from build123d import *

# Parameters (mm, degrees)
F0_W     = 11.7
F0_H     = 4
F1_DEPTH = 88.9
F3_DEPTH = 25
F4_R     = 0.5
F5_DEPTH = 25
F6_R     = 1
F7_DEPTH = 12.701
F13_R    = 0.5


with BuildPart() as f1:
    # F0 (on Top) → F1 (new body)
    with BuildSketch(Plane.XY):
        with BuildLine():
            Line((12.2, 0), (0.5, 0))
            ThreePointArc((0.5, 0), (0.1464466094, -0.1464466094), (0, -0.5))
            Line((0, -0.5), (0, -4.5))
            ThreePointArc((0, -4.5), (0.1464466094, -4.8535533906), (0.5, -5))
            Line((0.5, -5), (12.2, -5))
            ThreePointArc((12.2, -5), (12.5535533906, -4.8535533906), (12.7, -4.5))
            Line((12.7, -4.5), (12.7, -0.5))
            ThreePointArc((12.7, -0.5), (12.5535533906, -0.1464466094), (12.2, 0))
        make_face()
        with Locations((6.35, -2.5)):
            Rectangle(F0_W, F0_H, mode=Mode.SUBTRACT)
    extrude(amount=F1_DEPTH)

    # F2 (on face) → F3 (cut)
    with BuildSketch(Plane.XZ.offset(5)):
        Polygon((3.7468838188, 3.0342543032), (1.7641486272, 0), (10.9358513728, 0), (8.9531161812, 3.0342543032), (6.35, 3.0342543032), align=None)
    extrude(amount=-F3_DEPTH, mode=Mode.SUBTRACT)

    # F4 (on face) → F5 (cut)
    with BuildSketch(Plane(origin=(0, 0, 0), x_dir=(-1, 0, 0), z_dir=(0, 1, 0))):
        with Locations((-6.35, 17.8078599274)):
            Circle(F4_R)
    extrude(amount=-F5_DEPTH, mode=Mode.SUBTRACT)

    # F6 (on face) → F7 (cut, through all)
    with BuildSketch(Plane.YZ.offset(12.7)):
        with Locations((-2.5, 17.5)):
            Circle(F6_R)
    extrude(amount=-F7_DEPTH, mode=Mode.SUBTRACT)

    # F9 (on offset) → F10 (revolve)
    with BuildSketch(Plane.XY.offset(17.5)):
        Polygon((0.5120678688, -1.5), (0, -1.5), (0.1683332375, -2.5), (0.6804011064, -2.5), align=None)
    revolve(axis=Axis((0.6804011064, -2.5, 17.5), (1, 0, 0)))

    # F12: F1 across plane


with BuildPart() as f1_1:
    add(f1.part)
    add(f1.part.mirror(Plane(origin=(6.35, -2.5, 44.6902153566), x_dir=(0, 1, 0), z_dir=(1, 0, 0))))

    # F13
    f13_edges = [f1_1.edges().sort_by_distance(p)[0] for p in [
        (12.2, -4.5, 44.45),
        (0.5, -4.5, 44.45),
        (0.5, -0.5, 44.45),
        (12.2, -0.5, 44.45),
    ]]
    fillet(f13_edges, radius=F13_R)


solid = f1_1.part
Check sheet for the modelled part. Datum: model origin and axes. Units: mm. A direction names the side the tool comes from. Give positions to 0.01 mm unless a question says otherwise; leave off trailing zeros. Write each loop counter-clockwise with the first axis right and the second up, starting at its lowest first coordinate (ties: lowest second). Pieces come first, ordered by that corner, then holes. Notation, with made-up numbers: M -39.75,24.25 L -2.75,24.25 A27 ccw -2.75,40.25 Z; hole C 71,-8.75 d11. An arc over 180 degrees is marked long. Use one line per item in the form item = value.
(1) Draft check along Y on faces 1 (the flat face through (9.958, -0.253, 1.496)), 2 (the conical face through (12.03, -2.47, 17.44)), 3 (the flat face through (0.5, -3, 44)), 4 (the flat face through (6, 0, 44)). Enter one of: pulls with the +Y half, pulls with the -Y half, needs draft (parallel to the pull), parting line crosses it, or undercut.
Answer block:
face_1 = needs draft
face_2 = undercut
face_3 = undercut
face_4 = pulls with the +Y half
(2) Section check B-B on x = 10. Record the boundary of the cut face in (y, z).
Answer block:
outline = M -5,1.43 L -4.5,1.43 L -4.5,88.9 L -5,88.9 Z; M -0.5,1.43 L 0,1.43 L 0,88.9 L -0.5,88.9 Z
(3) Section check A-A on z = 15. Record the boundary of the cut face in (x, y).
Answer block:
outline = M 0,-4.5 A0.5 ccw 0.5,-5 L 12.2,-5 A0.5 ccw 12.7,-4.5 L 12.7,-0.5 A0.5 ccw 12.2,0 L 0.5,0 A0.5 ccw 0,-0.5 Z; hole M 0.5,-4 A0.5 ccw 1,-4.5 L 11.7,-4.5 A0.5 ccw 12.2,-4 L 12.2,-1 A0.5 ccw 11.7,-0.5 L 1,-0.5 A0.5 ccw 0.5,-1 Z
(4) Material ranges on line 1 along Z through (x, y) = (6.35, -0.15); line 2 along Y through (x, z) = (9.75, 55.5); line 3 along X through (y, z) = (-3.55, 17), recorded low to high.
Answer block:
line_1 = 3.03 to 17.31, 18.31 to 88.9
line_2 = -5 to -4.5, -0.5 to 0
line_3 = 0 to 0.5, 12.2 to 12.7
(5) Tool access check on faces 5 (the conical face through (0.67, -2.47, 17.44)), 6 (the flat face through (6.3, -4.7, 88.9)), 7 (the flat face through (6, -5, 44)), 8 (the flat face through (6, -4.5, 44)), 9 (the flat face through (9.958, -4.754, 1.496)). Record the directions out of +Z, -Z, +X, -X, +Y, -Y that give a thin tool (end or side, any length) a straight path to the whole face; none if there is none.
Answer block:
face_5 = none
face_6 = +Z, +X, -X, +Y, -Y
face_7 = +Z, -Z, +X, -X, -Y
face_8 = +Z, -Z
face_9 = -Z, +Y, -Y
(6) Depth check by flat-ended pin: P1, Ø3, axis at x = 7.5, y = -4, coming from the -Z side. Enter the tip coordinate at first touch or a pass-through.
Answer block:
P1 = 3.03
